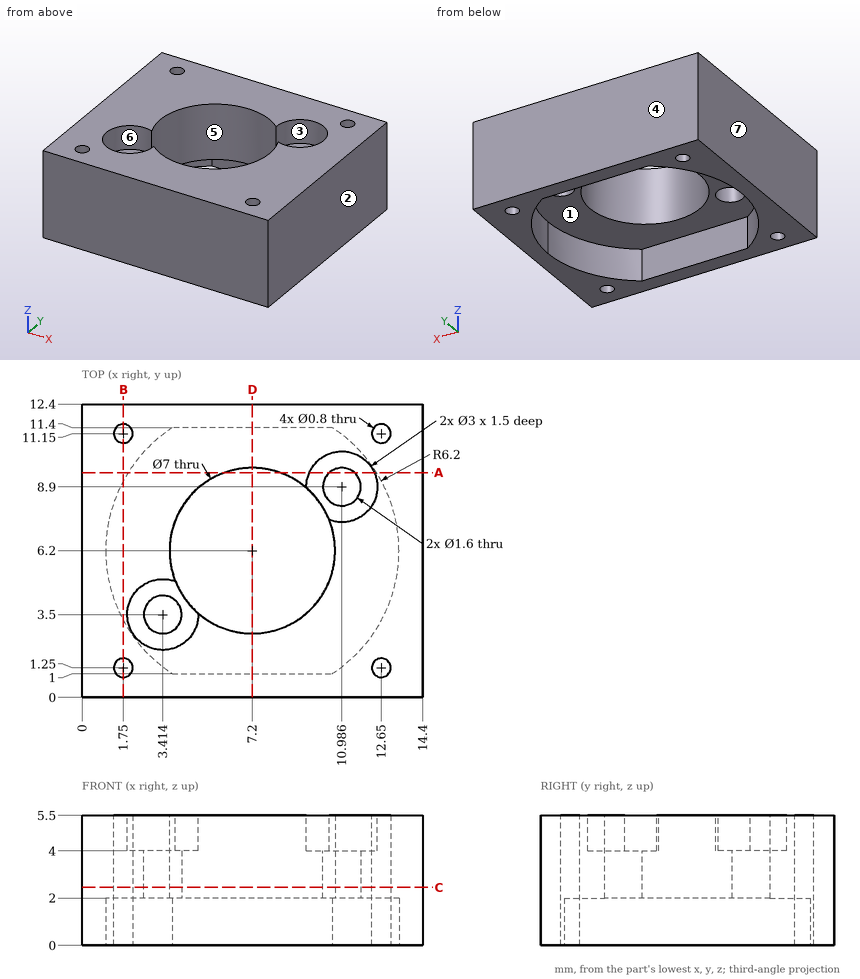
Geometry check sheet. Reference: drawing and pictorial views, mm from the part's lowest x, y, z. A direction names the side the tool comes from. Give positions to 0.01 mm unless a question says otherwise; leave off trailing zeros. Write each loop counter-clockwise with the first axis right and the second up, starting at its lowest first coordinate (ties: lowest second). Pieces come first, ordered by that corner, then holes. Notation, with made-up numbers: (-2, 2) -> (30, 2) arc R24 ccw to (30, 38) -> close; hole circle Ø9 at (45.5, -20.5). An arc over 180 degrees is marked (long way). One line per item, written item: value. Start each with the question number.
Item 1: Draft check along X on the marked faces 4, 5, 6 and 7. Enter one of: +X half, -X half, draft (parallel to the pull), parting line (faces both ways), or undercut.
Item 2: Section check C-C on z = 2.45. Record the cut outline in (x, y), then the cut area to 3 significant figures.
Item 3: Gauge pin test, flat ends, axial feed: pin 1 (5 mm diameter, centred on x = 6.5, y = 8.5, fed in from -Z); pin 2 (1.3 mm diameter, centred on x = 3.41, y = 3.5, fed in from +Z); pin 3 (1.5 mm diameter, centred on x = 4, y = 4, fed in from +Z). Record the tip position at first contact, or that the pin passes through.
Item 4: Material ranges on probe 1 along Y at (x, z) = (1.75, 3.5); probe 2 along Y at (x, z) = (6.5, 1.2); probe 3 along X at (y, z) = (1, 3.8), recorded low to high. Write a range as from..to.
Item 5: Tool access check on the marked faces 1, 2 and 3. Record the directions out of +Z, -Z, +X, -X, +Y, -Y that give a thin tool (end or side, any length) a straight path to the whole face; none if there is none.
Item 6: Section check A-A on y = 9.5. Record the cut outline in (x, z) (1 decimal).
Item 7: Section check D-D on x = 7.2. Record the cut outline in (y, z).
Item 8: Section check B-B on x = 1.75. Record the cut outline in (y, z), then the cut area to 3 significant figures.
Results list:
1. face 4: draft
1. face 5: undercut
1. face 6: undercut
1. face 7: -X half
2. outline: (0, 0) -> (14.4, 0) -> (14.4, 12.4) -> (0, 12.4) -> close; hole circle Ø0.8 at (1.75, 1.25); hole circle Ø0.8 at (1.75, 11.15); hole circle Ø1.6 at (3.41, 3.5); hole circle Ø7 at (7.2, 6.2); hole circle Ø1.6 at (10.99, 8.9); hole circle Ø0.8 at (12.65, 1.25); hole circle Ø0.8 at (12.65, 11.15)
2. area: 134 mm²
3. pin 1: z = 2
3. pin 2: through
3. pin 3: z = 4
4. probe 1: 0..0.85, 1.65..10.75, 11.55..12.4
4. probe 2: 0..1, 11.4..12.4
4. probe 3: 0..1.44, 2.06..12.34, 12.96..14.4
5. face 1: -Z
5. face 2: +Z, -Z, +X, +Y, -Y
5. face 3: +Z
6. outline: (0, 0) -> (2, 0) -> (2, 2) -> (6, 2) -> (6, 5.5) -> (0, 5.5) -> close; (8.4, 2) -> (10.5, 2) -> (10.5, 4) -> (9.6, 4) -> (9.6, 5.5) -> (8.4, 5.5) -> close; (11.5, 2) -> (12.4, 2) -> (12.4, 0) -> (14.4, 0) -> (14.4, 5.5) -> (12.4, 5.5) -> (12.4, 4) -> (11.5, 4) -> close
7. outline: (0, 0) -> (1, 0) -> (1, 2) -> (2.7, 2) -> (2.7, 5.5) -> (0, 5.5) -> close; (9.7, 2) -> (11.4, 2) -> (11.4, 0) -> (12.4, 0) -> (12.4, 5.5) -> (9.7, 5.5) -> close
8. outline: (0, 0) -> (0.85, 0) -> (0.85, 5.5) -> (0, 5.5) -> close; (1.65, 0) -> (3.24, 0) -> (3.24, 2) -> (9.16, 2) -> (9.16, 0) -> (10.75, 0) -> (10.75, 5.5) -> (1.65, 5.5) -> close; (11.55, 0) -> (12.4, 0) -> (12.4, 5.5) -> (11.55, 5.5) -> close
8. area: 47.6 mm²
